Model file for the job. Use its own axes, mm. Face numbers are marked on the shaded views. A direction names the side the tool comes from. Coordinates: 2 decimals unless noted, no trailing zeros. Write each loop counter-clockwise with the first axis right and the second up, starting at its lowest first coordinate (ties: lowest second). Pieces come first, ordered by that corner, then holes. Notation, with made-up numbers: M 75.25,-25.75 L 99.25,-25.75 A28 ccw 99.25,-4.75 Z; hole C 16,0 d1. An arc over 180 degrees is marked long. Put each result on its own line as item: value. Start each with the question number.
Q1. Drop flat-ended pins along their axis: pin 1 (5 mm diameter, centred on x = -8.5, y = 12.5, fed in from +Z); pin 2 (2 mm diameter, centred on y = 14.5, z = -2.5, fed in from +X); pin 3 (5 mm diameter, centred on x = -10, y = 13.5, fed in from +Z). Give the stop position or say it passes through.
Q2. Drill centre lines: line 1 along Z through (x, y) = (0, 2) (1 decimal); line 2 along Z through (x, y) = (0, 10). Where is each one in solid material? Low to high.
Q3. Which spindle directions (+Z, -Z, +X, -X, +Y, -Y) get a long thin tool onto all of the face, cutting with end or side? Do the marked faces 1 and 2. Say none if no direction does.
Q4. Pull direction X, two halves, no side cores. Call the marked faces 3, 4, 5 and 6: pulls with the +X half, pulls with the -X half, needs draft (parallel to the pull), parting line crosses it, or undercut.
Q5. Cut at D-D (y = 10.25). Write the cut outline in (x, z) (1 decimal).
Autodesk Inventor part; units mm, degrees
ref_plane "YZ Plane" through (0, 0, 0) normal (1, 0, 0) x (0, 1, 0)
ref_plane "XZ Plane" through (0, 0, 0) normal (0, 1, 0) x (-1, 0, 0)
ref_plane "XY Plane" through (0, 0, 0) normal (0, 0, 1) x (1, 0, 0)
sketch "Sketch1" plane through (0, 0, 0) normal (0, 1, 0) x (-1, 0, 0)
  line L0 (0, -20.0025) -> (0, 20.0025)
  line L1 (-20.0025, 0) -> (20.0025, 0)
  circle A0 centre (0, 0) radius 14.2875
  dimension "d0" = 28.575
extrude "Extrusion1" add sketch "Sketch1" along normal blind 19.05
sketch "Sketch2" plane through (0, 19.05, 0) normal (0, 1, 0) x (1, 0, 0)
  line L0 (0, 20.0025) -> (0, -20.0025)
  line L1 (20.0025, 0) -> (-20.0025, 0)
  point P0 (0, 0)
sketch "Sketch3" plane through (0, 19.05, 0) normal (0, 1, 0) x (1, 0, 0)
  point P0 (0, 0)
hole "Hole1" at (0, 19.05, 0) direction (0, -1, 0) diameter 6.35 end through all counterbore diameter 18.288 counterbore depth 12.7
chamfer "Chamfer1" distance 1.27 angle 45 1 edges at (0, 19.05, -9.144)
properties material "ABS, BEIGE"
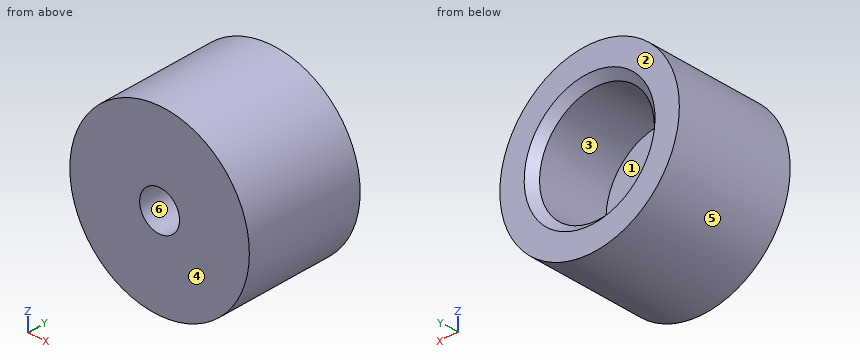
Computed values:
1. pin 1: z = 12.97
1. pin 2: x = 14.21
1. pin 3: z = 12.16
2. line 1: -14.3 to -3.2, 3.2 to 14.3
2. line 2: -14.29 to -9.14, 9.14 to 14.29
3. face 1: +Y
3. face 2: +Z, -Z, +X, -X, +Y
4. face 3: undercut
4. face 4: needs draft
4. face 5: parting line crosses it
4. face 6: undercut
5. outline: C 0,0 d28.6; hole C 0,0 d18.3
